from build123d import *

# Parameters (mm, degrees)
BOSS_EXTRUDE1_DEPTH = 20
LOFT1_START         = -34.8
LOFT1_DEPTH         = 69.6
LOFT1_START_2       = -28
LOFT1_2_DEPTH       = 56
BOSS_EXTRUDE2_START = -2
BOSS_EXTRUDE2_DEPTH = 50
BOSS_EXTRUDE3_DEPTH = 2.3
BOSS_EXTRUDE4_DEPTH = 2.3
CUT_EXTRUDE1_START  = -69.6
SKETCH7_R           = 5.3
CUT_EXTRUDE1_DEPTH  = 2
CUT_EXTRUDE2_DEPTH  = 70


with BuildPart() as part:
    # Sketch1 → Boss-Extrude1 (new body)
    with BuildSketch(Plane(origin=(0, 0, 0), x_dir=(1, 0, 0), z_dir=(0, 1, 0))):
        Polygon((27, 34.8), (-27, 34.8), (-27, 0), (-27, -34.8), (27, -34.8), (27, 0), align=None)
        Polygon((25, 0), (25, 32.8), (-25, 32.8), (-25, 0), (-25, -32.8), (25, -32.8), align=None, mode=Mode.SUBTRACT)
    extrude(amount=BOSS_EXTRUDE1_DEPTH)

    # Loft1: read off the stored shape, not the designer's step
    # Loft1 outline → Loft1 (add)
    with BuildSketch(Plane.XY.offset(LOFT1_START)):
        Polygon((-27, 20), (27, 20), (25, 35), (-25, 35), align=None)
    extrude(amount=LOFT1_DEPTH)

    # Loft1 2 outline → Loft1 2 (cut)
    with BuildSketch(Plane.YZ.offset(LOFT1_START_2)):
        Polygon((20, 34.8), (35, 32.8), (35, 34.8), align=None)
        Polygon((35, -32.8), (20, -34.8), (35, -34.8), align=None)
    extrude(amount=LOFT1_2_DEPTH, mode=Mode.SUBTRACT)

    # Cut-Loft1: read off the stored shape, not the designer's step
    # Cut-Loft1: loft between two sections, ruled curve by curve
    cut_loft1_from = [
        Edge.make_line((-25, 20, 32.8), (-25, 20, -32.8)),
        Edge.make_line((-25, 20, -32.8), (25, 20, -32.8)),
        Edge.make_line((25, 20, 32.8), (-25, 20, 32.8)),
        Edge.make_line((25, 20, -32.8), (25, 20, 32.8)),
    ]
    cut_loft1_to = [
        Edge.make_line((-23, 35, 30.8), (-23, 35, -30.8)),
        Edge.make_line((-23, 35, -30.8), (23, 35, -30.8)),
        Edge.make_line((23, 35, 30.8), (-23, 35, 30.8)),
        Edge.make_line((23, 35, -30.8), (23, 35, 30.8)),
    ]
    cut_loft1 = Solid(Shell([*[Face.make_surface_from_curves(cut_loft1_from[k], cut_loft1_to[k]) for k in range(4)], Face(Wire(cut_loft1_from)), Face(Wire(cut_loft1_to))]))
    add(cut_loft1, mode=Mode.SUBTRACT)

    # Sketch2 → Boss-Extrude2 (add)
    with BuildSketch(Plane(origin=(27, 0, 0), x_dir=(0, 0, -1), z_dir=(1, 0, 0)).offset(BOSS_EXTRUDE2_START)):
        with BuildLine():
            Line((32.8, 35), (32.8, 38.5))
            ThreePointArc((32.8, 38.5), (32.653553391, 38.853553391), (32.3, 39))
            Line((32.3, 39), (29.6, 39))
            ThreePointArc((29.6, 39), (29.246446609, 38.853553391), (29.1, 38.5))
            Line((29.1, 38.5), (29.1, 37.468550682))
            ThreePointArc((29.1, 37.468550682), (29.138060234, 37.277208966), (29.246446609, 37.114997291))
            Line((29.246446609, 37.114997291), (31.361443901, 35))
            Line((31.361443901, 35), (32.8, 35))
        make_face()
    extrude(amount=-BOSS_EXTRUDE2_DEPTH)

    # Sketch7 → Cut-Extrude1 (cut)
    with BuildSketch(Plane.XY.offset(34.8).offset(CUT_EXTRUDE1_START)):
        with Locations((0, 10)):
            Circle(SKETCH7_R)
    extrude(amount=CUT_EXTRUDE1_DEPTH, mode=Mode.SUBTRACT)

    # Sketch8 → Cut-Extrude2 (cut)
    with BuildSketch(Plane.ZY.offset(27)):
        with BuildLine():
            Line((-25.8, 6), (-22.8, 6))
            ThreePointArc((-22.8, 6), (-21.8, 4), (-22.8, 2))
            Line((-22.8, 2), (-25.8, 2))
            ThreePointArc((-25.8, 2), (-26.8, 4), (-25.8, 6))
        make_face()
        with BuildLine():
            Line((22.8, 6), (25.8, 6))
            ThreePointArc((25.8, 6), (26.8, 4), (25.8, 2))
            Line((25.8, 2), (22.8, 2))
            ThreePointArc((22.8, 2), (21.8, 4), (22.8, 6))
        make_face()
    extrude(amount=-CUT_EXTRUDE2_DEPTH, mode=Mode.SUBTRACT)


with BuildPart() as body_2:
    # Sketch5 → Boss-Extrude3 (new body)
    with BuildSketch(Plane.XZ):
        with BuildLine():
            Line((-25, -34.8), (-25, -9.8))
            ThreePointArc((-25, -9.8), (0, 15.2), (25, -9.8))
            Line((25, -9.8), (25, -34.8))
            Line((25, -34.8), (27, -34.8))
            Line((27, -34.8), (27, 34.8))
            Line((27, 34.8), (-27, 34.8))
            Line((-27, 34.8), (-27, -34.8))
            Line((-27, -34.8), (-25, -34.8))
        make_face()
    extrude(amount=BOSS_EXTRUDE3_DEPTH)

    # Sketch6 → Boss-Extrude4 (add)
    with BuildSketch(Plane.XZ.offset(2.3)):
        with BuildLine():
            Line((22.7, -34.8), (27, -34.8))
            Line((27, -34.8), (27, 34.8))
            Line((27, 34.8), (-27, 34.8))
            Line((-27, 34.8), (-27, -34.8))
            Line((-27, -34.8), (-22.7, -34.8))
            Line((-22.7, -34.8), (-22.7, -9.8))
            ThreePointArc((-22.7, -9.8), (0, 12.9), (22.7, -9.8))
            Line((22.7, -9.8), (22.7, -34.8))
        make_face()
    extrude(amount=BOSS_EXTRUDE4_DEPTH)


solid = part.part
Verification items for the finished model (mm, model axes). A direction names the side the tool comes from. Coordinates: 2 decimals unless noted, no trailing zeros. Order: outer loops, then holes, each group sorted by start corner. A loop starts at its lowest first (then second) coordinate and runs counter-clockwise, first axis right, second up. Notation, with made-up numbers: (33, 33.5) -> (69, 33.5) arc R32 cw to (69, 66.5) -> close; hole circle Ø2 at (46.5, -6.75). An arc over 180 degrees is marked (long way). Use CSV: the item, a comma, the result in double quotes. Start each with the question number.
Q1. Tool access check on faces 5 (the flat face through (26, 2, -24)), 6 (the flat face through (-25, 37, -31)), 7 (the flat face through (6, 10, -32.8)). Record the directions out of +Z, -Z, +X, -X, +Y, -Y that give a thin tool (end or side, any length) a straight path to the whole face; none if there is none.
Q2. Draft check along Z on faces 1 (the flat face through (0, 39, -31)), 2 (the flat face through (-0.378, 27.605, -33.786)), 3 (the cylindrical face through (26, 4, 26.8)), 4 (the flat face through (-26, 2, 24)). Enter one of: +Z half, -Z half, draft (parallel to the pull), parting line (faces both ways), or undercut.
Q3. Section check A-A, the plane y = 10. Record the cut outline in (x, z).
Q4. Section check B-B, the plane x = 0. Give the number of separate pieces and of enclosed holes in the cut face, and give its area (3 significant figures).
Q5. Depth check by flat-ended pin: P1, Ø3, axis at y = 37.5, z = -31.5, coming from the -X side; P2, Ø1.5, axis at x = 18, y = 33.5, coming from the +Z side; P3, Ø3, axis at y = 32.5, z = 26, coming from the +X side. Enter the tip coordinate at first touch or a pass-through.
Q6. Thickness scan on line 1 along Z through (x, y) = (-1.5, 19); line 2 along X through (y, z) = (15, 19); line 3 along Z through (x, y) = (-2.5, 37.5). Record the ranges inside material, lowest first.
Returned:
1,face 5,"+X, -X"
1,face 6,"+Z, -Z, -X, +Y"
1,face 7,"-Y"
2,face 1,"draft"
2,face 2,"-Z half"
2,face 3,"undercut"
2,face 4,"undercut"
3,outline,"(-27, -34.8) -> (-5.3, -34.8) -> (-5.3, -32.8) -> (-25, -32.8) -> (-25, 32.8) -> (25, 32.8) -> (25, -32.8) -> (5.3, -32.8) -> (5.3, -34.8) -> (27, -34.8) -> (27, 34.8) -> (-27, 34.8) -> close"
4,separate pieces,"3"
4,enclosed holes,"0"
4,area,"131 mm^2"
5,P1,"stops at x = -25"
5,P2,"stops at z = 33.1"
5,P3,"stops at x = 25.53"
6,line 1,"z = -34.8 to -32.8, 32.8 to 34.8"
6,line 2,"x = -27 to -25, 25 to 27"
6,line 3,"z = -32.8 to -29.1"
